Autodesk Inventor part; units mm, degrees
ref_plane "YZ Plane" through (0, 0, 0) normal (1, 0, 0) x (0, 1, 0)
ref_plane "XZ Plane" through (0, 0, 0) normal (0, 1, 0) x (-1, 0, 0)
ref_plane "XY Plane" through (0, 0, 0) normal (0, 0, 1) x (1, 0, 0)
sketch "Sketch1" plane through (0, 0, 0) normal (0, 0, 1) x (1, 0, 0)
  line L0 (20, 12.5) -> (20, -17.5)
  line L1 (20, -17.5) -> (-20, -17.5)
  line L2 (-20, -17.5) -> (-20, 12.5)
  circle A0 centre (-17.5, 12.5) radius 2.5
  circle A1 centre (17.5, 12.5) radius 2.5
  arc A2 (-15, 12.5) -> (15, 12.5) centre (0, 12.5) ccw
  point P0 (0, 0)
  dimension "d0" = 40
  dimension "d2" = 5
  dimension "d3" = 5
  dimension "d4" = 30
  dimension "d5" = 20
  dimension "d6" = 17.5
  dimension "d7" = 15
extrude "Extrusion1" add sketch "Sketch1" along normal blind 1.5 contours L0 L1 L2 A0 A2 A1
extrude "Extrusion2" add sketch "Sketch1" along normal blind 30 contours A1 | A0
fillet "Fillet1" radius 2.5 2 edges at (-20, 12.5, 30) (15, 12.5, 30)
sketch "Sketch2" plane through (0, 0, 0) normal (0, 0, 1) x (1, 0, 0)
  line L0 (-20, -17.5) -> (20, -17.5)
  line L1 (-20, -17.5) -> (20, -17.5)
  line L2 (-20, -17.5) -> (20, -17.5)
  line L3 (20, -17.5) -> (20, -19)
  line L4 (20, -19) -> (-20, -19)
  line L5 (-20, -19) -> (-20, -17.5)
  point P0 (0, 0)
  dimension "d13" = 1.5
extrude "Extrusion3" add sketch "Sketch2" along normal blind 120
sketch "Sketch5" plane through (-20, -17.5, 1.5) normal (0, 1, 0) x (1, 0, 0)
  line L0 (0, 0) -> (0, -118.5)
  line L1 (40, 0) -> (40, -118.5)
  line L2 (0, -81.0917) -> (40, -81.0917)
  line L3 (40, -81.0917) -> (40, -82.5917)
  line L4 (40, -82.5917) -> (0, -82.5917)
  line L5 (0, -82.5917) -> (0, -81.0917)
  line L6 (0, 0) -> (40, 0)
  point P0 (20, 1.5)
  point P1 (0, -82.5917)
  dimension "d25" = 1.5
  dimension "d26" = 81.0917
extrude "Extrusion5" add sketch "Sketch5" along normal blind 40 contours L2 L1 L4 L0
sketch "Sketch7" plane through (-20, -17.5, 84.0917) normal (0, 0, 1) x (1, 0, 0)
  arc A0 (9.6688, 20.825) -> (30.3312, 20.825) centre (20, 31.7) ccw
  line L0 (40, 0) -> (0, 0)
  line L1 (40, 0) -> (0, 0)
  line L2 (0, 0) -> (1.2374, 17.5516)
  arc A1 (9.6688, 20.825) -> (1.2374, 17.5516) centre (6.225, 17.2) ccw
  line L3 (40, 0) -> (38.7626, 17.5516)
  arc A2 (38.7626, 17.5516) -> (30.3312, 20.825) centre (33.775, 17.2) ccw
  line L4 (20, 0.597) -> (20, 58.4364) construction
  line L5 (40, 0) -> (40, 40)
  line L6 (40, 0) -> (40, 40)
  line L7 (0, 0) -> (0, 40)
  line L8 (40, 40) -> (0, 40)
  line L9 (0, 40) -> (0, 0)
  point P0 (20, 17.5)
  dimension "d36" = 30
  dimension "d37" = 31.7
  dimension "d38" = 5
  dimension "d39" = 17.2
extrude "Extrusion7" cut sketch "Sketch7" against normal up to surface (1.5 mm away) contours A1 L2 L7 L8 L5 L3 A2 A0
equation "\"d2\" = arm_thickness"
equation "\"d3\" = arm_thickness"
equation "\"d4\" = top_prong_height"
equation "\"d7\" = 3 * arm_thickness"
equation "\"d8\" = material_thickness"
equation "\"d10\" = arm_length"
equation "\"d12\" = 0.5 * arm_thickness"
equation "\"d13\" = material_thickness"
equation "\"d25\" = material_thickness"
equation "\"d36\" = handle_cutout_radius"
equation "\"d37\" = top_prong_height + prong_handle_height"
equation "\"arm_thickness\" = 5"
equation "\"material_thickness\" = 1.5"
equation "\"arm_length\" = 30"
equation "\"top_prong_height\" = 30"
equation "\"handle_cutout_radius\" = 30"
equation "\"prong_handle_height\" = 1.7"
properties part number "my_portafilter_holder_23ipt"
Geometry: final body of the model. Coordinates: model frame, mm. A direction names the side the tool comes from. Coordinates: 2 decimals unless noted, no trailing zeros. Write each loop counter-clockwise with the first axis right and the second up, starting at its lowest first coordinate (ties: lowest second). Pieces come first, ordered by that corner, then holes. Notation, with made-up numbers: (18, -11) - (68, -11) arc R14 ccw to (68, 12) - close; hole circle Ø2 at (22, -4.5). An arc over 180 degrees is marked (long way). Return JSON: item names as keys, results as strings.
Item 1: Reachability of faces 5 (the face through (15.66, 4.33, 83.35)), 6 (the face through (0, -17.5, 102)), 7 (the face through (-18.04, 14.94, 13.56)) from +Z, -Z, +X, -X, +Y, -Y: full face, straight path, thin tool, end or side. Return the list, or none.
Completed:
{"face 5": "+Z, +Y", "face 6": "+Z, +X, -X, +Y", "face 7": "+Z"}
Item 2: Section query D-D (y = -9). Output: boundary loops of the cut face in (x, z), and give its area (3 significant figures).
Completed:
{"outline": "(-20, 0) - (20, 0) - (20, 1.5) - (-20, 1.5) - close; (-19.4, 82.59) - (19.4, 82.59) - (19.4, 84.09) - (-19.4, 84.09) - close", "area": "118 mm2"}
Item 3: Line query: L1, parallel to Z at x = -15, y = -2; L2, parallel to Y at x = 6, z = 39; L3, parallel to X at y = -11.5, z = 83. Output: solid intervals per line, ascending.
Completed:
{"L1": "z = 0 to 1.5, 82.59 to 84.09", "L2": "y = -19 to -17.5", "L3": "x = -19.58 to 19.58"}
Item 4: Pull-direction query (X, two-part tool) for faces 1 (the face through (20, -18, 60)), 2 (the face through (-20, -18, 60)), 3 (the face through (0, -9, 82.592)), 4 (the face through (0.33, -2.496, 0.74)); classes: +X half, -X half, draft (parallel to the pull), parting line (faces both ways), or undercut.
Completed:
{"face 1": "+X half", "face 2": "-X half", "face 3": "draft", "face 4": "undercut"}
Item 5: Section query B-B (z = 8.5). Output: boundary loops of the cut face in (x, y), and give its area (3 significant figures).
Completed:
{"outline": "(-20, -19) - (20, -19) - (20, -17.5) - (-20, -17.5) - close; circle Ø5 at (-17.5, 12.5); circle Ø5 at (17.5, 12.5)", "area": "99.3 mm2"}
Item 6: Pin query (flat end, axial travel): pin 1 Ø3 at (x, z) = (11, 50.5) entering from +Y; pin 2 Ø11 at (x, y) = (2, -7) entering from +Z. Return the tip coordinate at first contact, or that it passes through.
Completed:
{"pin 1": "stops at y = -17.5", "pin 2": "stops at z = 84.09"}
Item 7: Section query A-A (y = -4). Output: boundary loops of the cut face in (x, z), and give its area (3 significant figures).
Completed:
{"outline": "(-20, 0) - (20, 0) - (20, 1.5) - (-20, 1.5) - close; (-19.05, 82.59) - (19.05, 82.59) - (19.05, 84.09) - (-19.05, 84.09) - close", "area": "117 mm2"}
Item 8: Section query C-C (x = -17.5). Output: boundary loops of the cut face in (y, z), and give its area (3 significant figures).
Completed:
{"outline": "(-19, 0) - (15, 0) - (15, 27.5) arc R2.5 ccw to (10, 27.5) - (10, 1.5) - (-17.5, 1.5) - (-17.5, 82.59) - (3.04, 82.59) - (3.04, 84.09) - (-17.5, 84.09) - (-17.5, 120) - (-19, 120) - close", "area": "399 mm2"}
